```python
from build123d import *

# Parameters (mm, degrees)
F0_W     = 27.764633
F0_H     = 7.2
F1_DEPTH = 2
F2_R     = 1
F3_SIZE  = 0.5
F4_SIZE  = 0.4


with BuildPart() as f1:
    # F0 (on Top) → F1 (new body)
    with BuildSketch(Plane.XY):
        with Locations((9.957446, 0)):
            Rectangle(F0_W, F0_H)
        Polygon((2.424871, 0), (1.212436, -2.1), (-1.212436, -2.1), (-2.424871, 0), (-1.212436, 2.1), (1.212436, 2.1), align=None, mode=Mode.SUBTRACT)
        Polygon((7.619913, 0), (6.696152, -1.6), (4.848632, -1.6), (3.924871, 0), (4.848632, 1.6), (6.696152, 1.6), align=None, mode=Mode.SUBTRACT)
        Polygon((12.848198, 0), (12.068775, -1.35), (10.50993, -1.35), (9.730507, 0), (10.50993, 1.35), (12.068775, 1.35), align=None, mode=Mode.SUBTRACT)
        Polygon((17.762655, 0), (17.12757, -1.1), (15.857399, -1.1), (15.222314, 0), (15.857399, 1.1), (17.12757, 1.1), align=None, mode=Mode.SUBTRACT)
        Polygon((22.339762, 0), (21.849014, -0.85), (20.867519, -0.85), (20.376771, 0), (20.867519, 0.85), (21.849014, 0.85), align=None, mode=Mode.SUBTRACT)
    extrude(amount=F1_DEPTH)

    # F2
    f2_edges = [f1.edges().sort_by_distance(p)[0] for p in [
        (-3.924871, -3.6, 1),
        (23.839762, -3.6, 1),
        (23.839762, 3.6, 1),
        (-3.924871, 3.6, 1),
    ]]
    fillet(f2_edges, radius=F2_R)

    # F3
    f3_edges = [f1.edges().sort_by_distance(p)[0] for p in [
        (9.957445, -3.6, 0),
        (9.957445, -3.6, 2),
    ]]
    chamfer(f3_edges, length=F3_SIZE)

    # F4
    f4_edges = [f1.edges().sort_by_distance(p)[0] for p in [
        (-1.818653, -1.05, 2),
        (-1.818653, 1.05, 2),
        (0, 2.1, 2),
        (1.818653, 1.05, 2),
        (1.818653, -1.05, 2),
        (0, -2.1, 2),
        (4.386751, -0.8, 2),
        (4.386751, 0.8, 2),
        (5.772392, 1.6, 2),
        (7.158033, 0.8, 2),
        (7.158033, -0.8, 2),
        (5.772392, -1.6, 2),
        (11.289353, -1.35, 2),
        (10.120218, -0.675, 2),
        (10.120218, 0.675, 2),
        (11.289353, 1.35, 2),
        (12.458487, 0.675, 2),
        (12.458487, -0.675, 2),
        (15.539857, -0.55, 2),
        (15.539857, 0.55, 2),
        (16.492485, 1.1, 2),
        (17.445113, 0.55, 2),
        (17.445113, -0.55, 2),
        (16.492485, -1.1, 2),
        (21.358266, -0.85, 2),
        (20.622145, -0.425, 2),
        (20.622145, 0.425, 2),
        (21.358266, 0.85, 2),
        (22.094388, 0.425, 2),
        (22.094388, -0.425, 2),
    ]]
    chamfer(f4_edges, length=F4_SIZE)


solid = f1.part
```
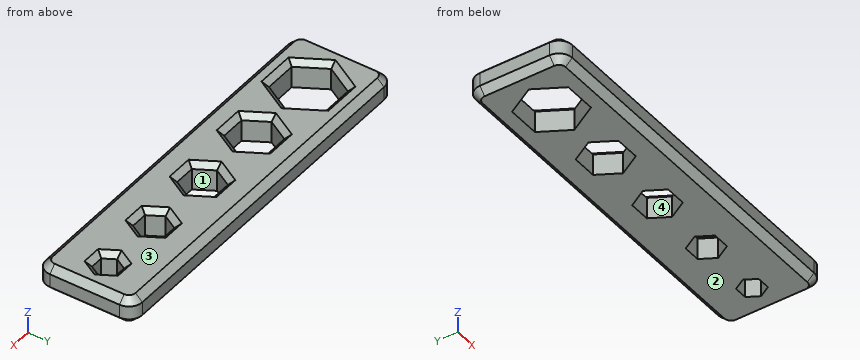
The model under review builds one solid part; all positions refer to its coordinate system, in mm. Face numbers are marked on the shaded views. A direction names the side the tool comes from. Give positions to 0.01 mm unless a question says otherwise; leave off trailing zeros. Write each loop counter-clockwise with the first axis right and the second up, starting at its lowest first coordinate (ties: lowest second). Pieces come first, ordered by that corner, then holes. Notation, with made-up numbers: M 36,25 L 45,25 A21 cw 45,36 Z; hole C -36.75,61 d8. An arc over 180 degrees is marked long. Answer in a Markdown table with one row per item.
Item 1: Draft analysis for pull direction Y (two halves, no side actions). For the marked faces 3 and 4, state which applies: +Y half, -Y half, draft (parallel to the pull), parting line (faces both ways), or undercut.
Check sheet entries:
| item | result |
|---|---|
| face 3 | draft |
| face 4 | undercut |
Item 2: For line 1 along Y through (x, z) = (12, 1.2); line 2 along X through (y, z) = (1.5, 0.1); line 3 along Y through (x, z) = (5, 1.2), list the stretches that pass through material, from the lowest coordinate up.
Check sheet entries:
| item | result |
|---|---|
| line 1 | -3.6 to -1.35, 1.35 to 3.6 |
| line 2 | -3.52 to -1.56, 1.56 to 4.79, 6.75 to 23.44 |
| line 3 | -3.6 to -1.6, 1.6 to 3.6 |
Item 3: Add section B-B on z = 0.85. State how many separate pieces and enclosed holes the cut face has, plus the area to 3 significant figures.
Check sheet entries:
| item | result |
|---|---|
| separate pieces | 1 |
| enclosed holes | 5 |
| area | 162 mm2 |
Item 4: Add section A-A on x = 11.75. Give the boundary of the cut face in (y, z).
Check sheet entries:
| item | result |
|---|---|
| outline | M -3.6,0.5 L -3.1,0 L -1.35,0 L -1.35,1.6 L -1.75,2 L -3.1,2 L -3.6,1.5 Z; M 1.35,0 L 3.1,0 L 3.6,0.5 L 3.6,1.5 L 3.1,2 L 1.75,2 L 1.35,1.6 Z |
Item 5: Tool access review of the marked faces 1 and 2: name each direction out of +Z, -Z, +X, -X, +Y, -Y from which nothing blocks a thin tool from reaching the whole face with its end or side.
Check sheet entries:
| item | result |
|---|---|
| face 1 | +Z, -Z |
| face 2 | -Z, +X, -X, +Y, -Y |
